The figure shows three views and two pictorial views of one solid part (mm, origin at its lowest corner). Answer the questions. A direction names the side the tool comes from. Give positions to 0.01 mm unless a question says otherwise; leave off trailing zeros. Write each loop counter-clockwise with the first axis right and the second up, starting at its lowest first coordinate (ties: lowest second). Pieces come first, ordered by that corner, then holes. Notation, with made-up numbers: (78, -15.5) - (83, -15.5) arc R12 cw to (83, -11.5) - close; hole circle Ø7 at (62, 54). An arc over 180 degrees is marked (long way). Use a Markdown table: item, result. Add a question column.
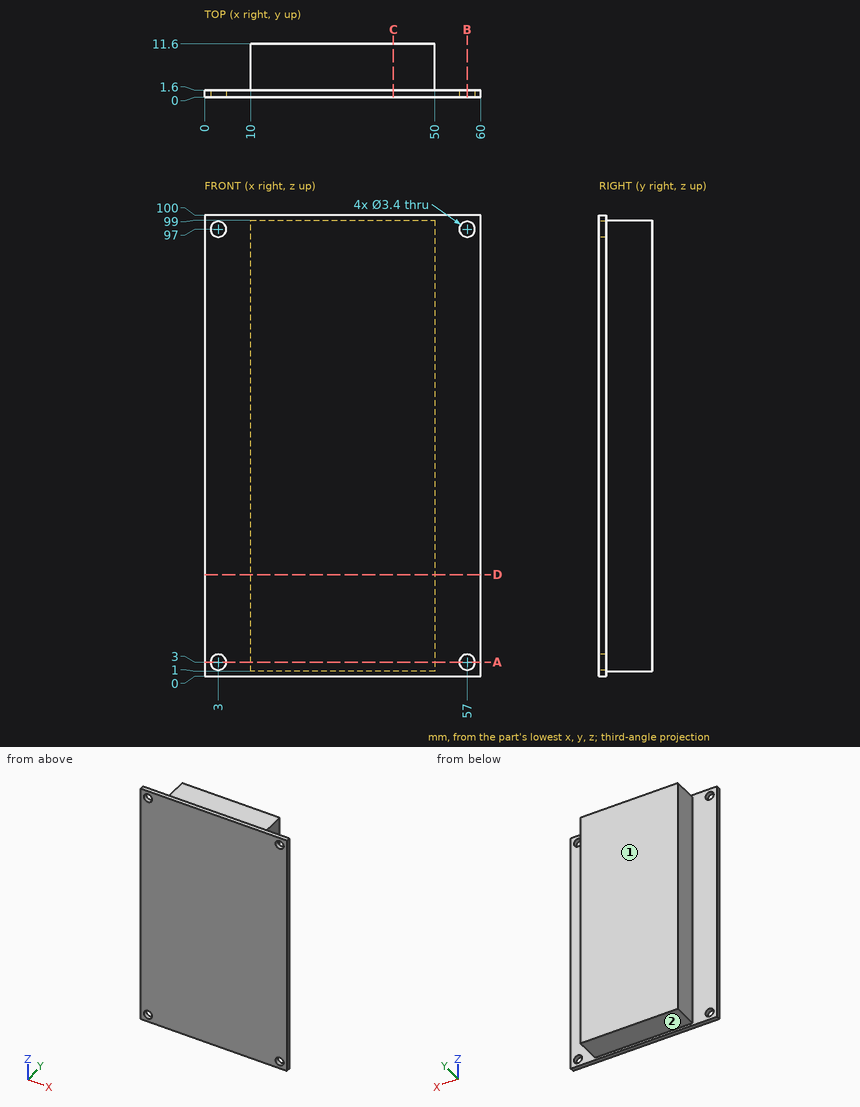
1. The part is cut by section B-B (x = 57). Give the vertices of the cut face in (y, z), and give its area (3 significant figures).
2. The part is cut by section A-A (z = 3). Give the vertices of the cut face in (x, y), and give its area (3 significant figures).
3. Given P1, Ø1, axis at x = 28.5, y = 3.5, coming from the +Z side; P2, Ø2, axis at y = 5.5, z = 63, coming from the -X side; P3, Ø5, axis at y = 5.5, z = 48.5, coming from the +X side; P4, Ø3, axis at x = 57, z = 3, coming from the +Y side, each flat-ended and moving along its own axis, determine where each tip first touches the part or whether it passes through.
4. Which of the six approach directions +Z, -Z, +X, -X, +Y, -Y give full straight-line access (tool end or side, diameter ignored) to the marked faces 1 and 2?
5. Consider L1, parallel to Z at x = 57, y = 0.85; L2, parallel to X at y = 0.35, z = 97; L3, parallel to Z at x = 37.5, y = 3.5. Determine where each line is inside the solid, lowest interval first. Write a range as [from, to].
6. The part is cut by section C-C (x = 41). Give the vertices of the cut face in (y, z).
7. The part is cut by section D-D (z = 22). Give the vertices of the cut face in (x, y), and give its area (3 significant figures).
Check values:
| question | item | result |
|---|---|---|
| 1 | outline | (0, 0) - (1.6, 0) - (1.6, 1.3) - (0, 1.3) - close; (0, 4.7) - (1.6, 4.7) - (1.6, 95.3) - (0, 95.3) - close; (0, 98.7) - (1.6, 98.7) - (1.6, 100) - (0, 100) - close |
| 1 | area | 149 mm2 |
| 2 | outline | (0, 0) - (1.3, 0) - (1.3, 1.6) - (0, 1.6) - close; (4.7, 0) - (55.3, 0) - (55.3, 1.6) - (50, 1.6) - (50, 11.6) - (10, 11.6) - (10, 1.6) - (4.7, 1.6) - close; (58.7, 0) - (60, 0) - (60, 1.6) - (58.7, 1.6) - close |
| 2 | area | 485 mm2 |
| 3 | P1 | stops at z = 99 |
| 3 | P2 | stops at x = 10 |
| 3 | P3 | stops at x = 50 |
| 3 | P4 | passes through |
| 4 | face 1 | +Z, -Z, +X, -X, +Y |
| 4 | face 2 | -Z, +X, -X, +Y |
| 5 | L1 | z = [0, 1.3], [4.7, 95.3], [98.7, 100] |
| 5 | L2 | x = [0, 1.3], [4.7, 55.3], [58.7, 60] |
| 5 | L3 | z = [1, 99] |
| 6 | outline | (0, 0) - (1.6, 0) - (1.6, 1) - (11.6, 1) - (11.6, 99) - (1.6, 99) - (1.6, 100) - (0, 100) - close |
| 7 | outline | (0, 0) - (60, 0) - (60, 1.6) - (50, 1.6) - (50, 11.6) - (10, 11.6) - (10, 1.6) - (0, 1.6) - close |
| 7 | area | 496 mm2 |
